```python
from build123d import *

# Parameters (mm, degrees)
SKETCH1_W           = 30
SKETCH1_H           = 30
BOSS_EXTRUDE1_DEPTH = 2


with BuildPart() as part:
    # Sketch1 → Boss-Extrude1 (new body)
    with BuildSketch(Plane(origin=(0, 0, 0), x_dir=(1, 0, 0), z_dir=(0, 1, 0))):
        Polygon((-78.598325024, 37.862631579), (-78.598325024, 23.862631579), (-28.598325024, 23.862631579), (1.401674976, 23.862631579), (51.401674976, 23.862631579), (51.401674976, 37.862631579), (31.401674976, 37.862631579), (31.401674976, 27.862631579), (-58.598325024, 27.862631579), (-58.598325024, 37.862631579), align=None)
        with Locations((-13.598325024, 8.862631579)):
            Rectangle(SKETCH1_W, SKETCH1_H)
    extrude(amount=BOSS_EXTRUDE1_DEPTH)


solid = part.part
```
The model under review builds one solid part; all positions refer to its coordinate system, in mm. Give positions to 0.01 mm unless a question says otherwise; leave off trailing zeros. Write each loop counter-clockwise with the first axis right and the second up, starting at its lowest first coordinate (ties: lowest second). Pieces come first, ordered by that corner, then holes. Notation, with made-up numbers: M 56,62 L 112,62 A22 cw 112,94 Z; hole C -40,11.25 d7. An arc over 180 degrees is marked long. Write item = value, one per line. Start each with the question number.
Q1. For line 1 (X direction, y = 0.2, z = -22); line 2 (X direction, y = 1.9, z = -34.5); line 3 (Z direction, x = -66, y = 0.2), list the stretches that pass through material, from the lowest coordinate up.
Q2. Clearance check with flat-ended pins moving along their axes: pin 1 (0.6 mm diameter, centred on y = 1, z = -15, fed in from -X); pin 2 (0.6 mm diameter, centred on x = 26.5, y = 1, fed in from +Z). State where each tip first meets the part, or that it passes through.
Q3. We need section C-C (x = 37). State the section outline as (y, z) points.
Q4. We need section A-A (z = -35). State the section outline as (x, y) points, plus the area to 3 significant figures.
Q5. We need section B-B (y = 0.7). State the section outline as (x, z) points.
Q6. We need section D-D (z = -1.5). State the section outline as (x, y) points.
Result set:
q1.line_1 = -28.6 to 1.4
q1.line_2 = -78.6 to -58.6, 31.4 to 51.4
q1.line_3 = -37.86 to -23.86
q2.pin_1 = -28.6
q2.pin_2 = -23.86
q3.outline = M 0,-37.86 L 2,-37.86 L 2,-23.86 L 0,-23.86 Z
q4.outline = M -78.6,0 L -58.6,0 L -58.6,2 L -78.6,2 Z; M 31.4,0 L 51.4,0 L 51.4,2 L 31.4,2 Z
q4.area = 80.0 mm2
q5.outline = M -78.6,-37.86 L -58.6,-37.86 L -58.6,-27.86 L 31.4,-27.86 L 31.4,-37.86 L 51.4,-37.86 L 51.4,-23.86 L 1.4,-23.86 L 1.4,6.14 L -28.6,6.14 L -28.6,-23.86 L -78.6,-23.86 Z
q6.outline = M -28.6,0 L 1.4,0 L 1.4,2 L -28.6,2 Z
